```python
from build123d import *

# Parameters (mm, degrees)
SKETCH1_W           = 15.9
SKETCH1_H           = 13.6
BOSS_EXTRUDE1_DEPTH = 21.2
CUT_EXTRUDE1_DEPTH  = 15.24


with BuildPart() as part:
    # Sketch1 → Boss-Extrude1 (new body)
    with BuildSketch(Plane.XY):
        with Locations((7.95, 6.8)):
            Rectangle(SKETCH1_W, SKETCH1_H)
    extrude(amount=-BOSS_EXTRUDE1_DEPTH)

    # Sketch2 → Cut-Extrude1 (cut)
    with BuildSketch(Plane.XY):
        Polygon((1.32, 12.19437295), (14.58, 12.19437295), (14.58, 4.57437295), (11.024, 4.57437295), (11.024, 2.66937295), (8.94, 2.66937295), (8.94, 1.39937295), (6.908, 1.39937295), (6.908, 2.66937295), (4.876, 2.66937295), (4.876, 4.57437295), (1.32, 4.57437295), align=None)
    extrude(amount=-CUT_EXTRUDE1_DEPTH, mode=Mode.SUBTRACT)


solid = part.part
```
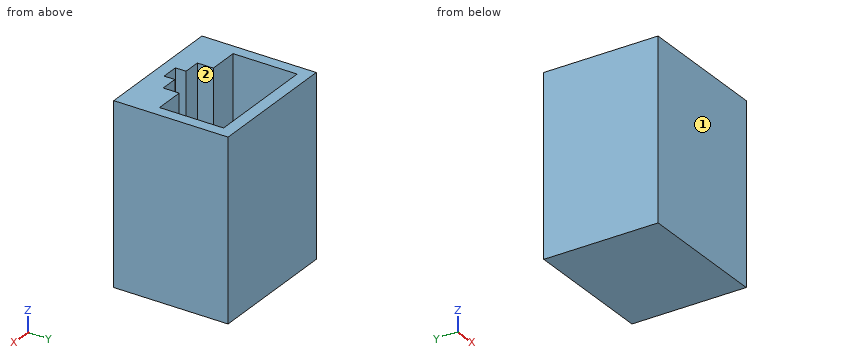
Verification items for the finished model (mm, model axes). Face numbers are marked on the shaded views. A direction names the side the tool comes from. Coordinates: 2 decimals unless noted, no trailing zeros. Order: outer loops, then holes, each group sorted by start corner. A loop starts at its lowest first (then second) coordinate and runs counter-clockwise, first axis right, second up. Notation, with made-up numbers: (-24.5, 63.25) - (-12.5, 63.25) arc R17 ccw to (-12.5, 84.25) - close; hole circle Ø7 at (9, -29). An arc over 180 degrees is marked (long way). Return JSON: item names as keys, results as strings.
(1) Section check A-A, the plane z = -3.25. Record the cut outline in (x, y), and give its area (3 significant figures).
Filled sheet:
{"outline": "(0, 0) - (15.9, 0) - (15.9, 13.6) - (0, 13.6) - close; hole (1.32, 4.57) - (4.88, 4.57) - (4.88, 2.67) - (6.91, 2.67) - (6.91, 1.4) - (8.94, 1.4) - (8.94, 2.67) - (11.02, 2.67) - (11.02, 4.57) - (14.58, 4.57) - (14.58, 12.19) - (1.32, 12.19) - close", "area": "101 mm^2"}
(2) Access from +Z, -Z, +X, -X, +Y, -Y to the whole of each face (thin tool, end or side, straight path). Record for the marked faces 1 and 2.
Filled sheet:
{"face 1": "+Z, -Z, +X, -X, -Y", "face 2": "+Z"}
(3) Section check C-C, the plane x = 3. Record the cut outline in (y, z), and give its area (3 significant figures).
Filled sheet:
{"outline": "(0, -21.2) - (13.6, -21.2) - (13.6, 0) - (12.19, 0) - (12.19, -15.24) - (4.57, -15.24) - (4.57, 0) - (0, 0) - close", "area": "172 mm^2"}
(4) Section check B-B, the plane y = 3. Record the cut outline in (x, z), and give its area (3 significant figures).
Filled sheet:
{"outline": "(0, -21.2) - (15.9, -21.2) - (15.9, 0) - (11.02, 0) - (11.02, -15.24) - (4.88, -15.24) - (4.88, 0) - (0, 0) - close", "area": "243 mm^2"}
(5) Thickness scan on line 1 along Y through (x, z) = (1.5, -14.75); line 2 along X through (y, z) = (1.5, -8.5); line 3 along X through (y, z) = (9.5, -15). Record the ranges inside material, lowest first.
Filled sheet:
{"line 1": "y = 0 to 4.57, 12.19 to 13.6", "line 2": "x = 0 to 6.91, 8.94 to 15.9", "line 3": "x = 0 to 1.32, 14.58 to 15.9"}
